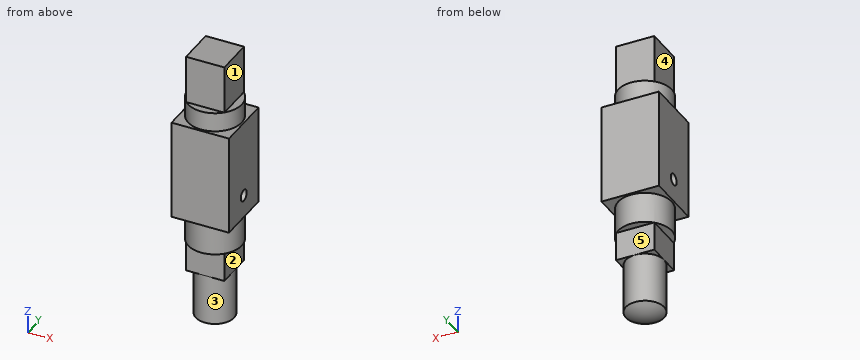
from build123d import *

# Parameters (mm, degrees)
SCHIZZO1_R                   = 5
ESTRUSIONE_ESTRUSIONE1_DEPTH = 13
SCHIZZO2_W                   = 10
SCHIZZO2_H                   = 10
ESTRUSIONE_ESTRUSIONE2_DEPTH = 7.5
SCHIZZO3_R                   = 7
ESTRUSIONE_ESTRUSIONE3_DEPTH = 8
SCHIZZO4_W                   = 15
SCHIZZO4_H                   = 15
ESTRUSIONE_ESTRUSIONE4_DEPTH = 26
SCHIZZO5_R                   = 7
ESTRUSIONE_ESTRUSIONE5_DEPTH = 5
SCHIZZO6_W                   = 10
SCHIZZO6_H                   = 10
ESTRUSIONE_ESTRUSIONE6_DEPTH = 12.5
CUPOLA1_FACE_RADIUS          = 5
CUPOLA1_HEIGHT               = 1.3
SCHIZZO7_R                   = 1.5
TAGLIO_ESTRUSIONE1_DEPTH     = 74.927329182


with BuildPart() as part:
    # Schizzo1 → Estrusione-Estrusione1 (new body)
    with BuildSketch(Plane.XY):
        with Locations(Location((0, 0, 0), (0, 0, 180))):
            Circle(SCHIZZO1_R)
    extrude(amount=ESTRUSIONE_ESTRUSIONE1_DEPTH)

    # Schizzo2 → Estrusione-Estrusione2 (add)
    with BuildSketch(Plane.XY.offset(13)):
        Rectangle(SCHIZZO2_W, SCHIZZO2_H)
    extrude(amount=ESTRUSIONE_ESTRUSIONE2_DEPTH)

    # Schizzo3 → Estrusione-Estrusione3 (add)
    with BuildSketch(Plane.XY.offset(20.5)):
        with Locations(Location((0, 0, 0), (0, 0, 135.584691403))):
            Circle(SCHIZZO3_R)
    extrude(amount=ESTRUSIONE_ESTRUSIONE3_DEPTH)

    # Schizzo4 → Estrusione-Estrusione4 (add)
    with BuildSketch(Plane.XY.offset(28.5)):
        Rectangle(SCHIZZO4_W, SCHIZZO4_H)
    extrude(amount=ESTRUSIONE_ESTRUSIONE4_DEPTH)

    # Schizzo5 → Estrusione-Estrusione5 (add)
    with BuildSketch(Plane.XY.offset(54.5)):
        with Locations(Location((0, 0, 0), (0, 0, 135.584691403))):
            Circle(SCHIZZO5_R)
    extrude(amount=ESTRUSIONE_ESTRUSIONE5_DEPTH)

    # Schizzo6 → Estrusione-Estrusione6 (add)
    with BuildSketch(Plane.XY.offset(59.5)):
        Rectangle(SCHIZZO6_W, SCHIZZO6_H)
    extrude(amount=ESTRUSIONE_ESTRUSIONE6_DEPTH)

    # Cupola1: a dome of height H over a round flat face of radius A is a cap of a sphere of radius (A * A + H * H) / (2 * H)
    cupola1_r = (CUPOLA1_FACE_RADIUS * CUPOLA1_FACE_RADIUS + CUPOLA1_HEIGHT * CUPOLA1_HEIGHT) / (2 * CUPOLA1_HEIGHT)
    cupola1_base = Plane((0, 0, 0), z_dir=(0, 0, -1))
    with Locations(cupola1_base.offset(CUPOLA1_HEIGHT - cupola1_r)):
        cupola1_ball = Sphere(cupola1_r, mode=Mode.PRIVATE)
    add(split(cupola1_ball, bisect_by=cupola1_base, keep=Keep.TOP, mode=Mode.PRIVATE))

    # Schizzo7 → Taglio-Estrusione1 (cut, through all)
    with BuildSketch(Plane.ZY.offset(7.5)):
        with Locations((34.5, 0)):
            Circle(SCHIZZO7_R)
    extrude(amount=-TAGLIO_ESTRUSIONE1_DEPTH, mode=Mode.SUBTRACT)


solid = part.part
Source: CAD feature listing. Evaluate the final solid. Frame: model axes, mm. Face numbers are marked on the shaded views. A direction names the side the tool comes from. Give positions to 0.01 mm unless a question says otherwise; leave off trailing zeros. Write each loop counter-clockwise with the first axis right and the second up, starting at its lowest first coordinate (ties: lowest second). Pieces come first, ordered by that corner, then holes. Notation, with made-up numbers: M 71.5,-40 L 110.5,-40 A32 ccw 110.5,-4 Z; hole C -27,-29 d11. An arc over 180 degrees is marked long. Return JSON: item names as keys, results as strings. Group by question number.
1) Cut plane A-A, the plane z = 34.5. Output: boundary loops of the cut face in (x, y).
2) Cut plane B-B, the plane y = 0.75. Output: boundary loops of the cut face in (x, z).
3) Set-up query: the marked faces 1, 2, 3, 4 and 5. Return all of +Z, -Z, +X, -X, +Y, -Y with unobstructed straight access to the full face (end or side cutting, diameter ignored); none if empty.
4) Cut plane C-C, the plane x = 4. Output: boundary loops of the cut face in (y, z), plus the area to 3 significant figures.
5) Pin query (flat end, axial travel): P1, Ø2, axis at y = 3, z = 62.5, coming from the -X side; P2, Ø2.5, axis at x = 2.5, y = -3, coming from the -Z side; P3, Ø8, axis at x = -3, y = 5, coming from the -Z side. Return the tip coordinate at first contact, or that it passes through.
6) Material intervals for line 1 along Y through (x, z) = (0.5, 62.5); line 2 along Z through (x, y) = (-5.5, 5.75); line 3 along X through (y, z) = (-1, 3), sorted ascending. Write a range as [from, to].
7) Cut plane D-D, the plane x = -3. Output: boundary loops of the cut face in (y, z), plus the area to 3 significant figures.
Recorded:
{
 "1": {"outline": "M -7.5,-7.5 L 7.5,-7.5 L 7.5,-1.5 L -7.5,-1.5 Z; M -7.5,1.5 L 7.5,1.5 L 7.5,7.5 L -7.5,7.5 Z"},
 "2": {"outline": "M -7.5,28.5 L -6.96,28.5 L -6.96,20.5 L -5,20.5 L -5,13 L -4.94,13 L -4.94,0 A10.24 ccw 4.94,0 L 4.94,13 L 5,13 L 5,20.5 L 6.96,20.5 L 6.96,28.5 L 7.5,28.5 L 7.5,33.2 L -7.5,33.2 Z; M -7.5,35.8 L 7.5,35.8 L 7.5,54.5 L 6.96,54.5 L 6.96,59.5 L 5,59.5 L 5,72 L -5,72 L -5,59.5 L -6.96,59.5 L -6.96,54.5 L -7.5,54.5 Z"},
 "3": {"face 1": "+Z, +X, +Y, -Y", "face 2": "-Z, +X, +Y, -Y", "face 3": "-Z", "face 4": "+Z, -X, +Y, -Y", "face 5": "-Z, +X, -X, +Y"},
 "4": {"outline": "M -7.5,28.5 L -5.74,28.5 L -5.74,20.5 L -5,20.5 L -5,13 L -3,13 L -3,0 A9.45 ccw 3,0 L 3,13 L 5,13 L 5,20.5 L 5.74,20.5 L 5.74,28.5 L 7.5,28.5 L 7.5,54.5 L 5.74,54.5 L 5.74,59.5 L 5,59.5 L 5,72 L -5,72 L -5,59.5 L -5.74,59.5 L -5.74,54.5 L -7.5,54.5 Z; hole C 0,34.5 d3", "area": "812 mm²"},
 "5": {"P1": "stops at x = -5", "P2": "stops at z = -0.95", "P3": "stops at z = -1.14"},
 "6": {"line 1": "y = [-5, 5]", "line 2": "z = [28.5, 54.5]", "line 3": "x = [-4.9, 4.9]"},
 "7": {"outline": "M -7.5,28.5 L -6.32,28.5 L -6.32,20.5 L -5,20.5 L -5,13 L -4,13 L -4,0 A9.82 ccw 4,0 L 4,13 L 5,13 L 5,20.5 L 6.32,20.5 L 6.32,28.5 L 7.5,28.5 L 7.5,54.5 L 6.32,54.5 L 6.32,59.5 L 5,59.5 L 5,72 L -5,72 L -5,59.5 L -6.32,59.5 L -6.32,54.5 L -7.5,54.5 Z; hole C 0,34.5 d3", "area": "856 mm²"}
}
